Read the model definition and answer for the solid it produces. Units are mm, in the model's axes. A direction names the side the tool comes from. Round coordinates to 2 decimals unless told otherwise and drop trailing zeros. Order: outer loops, then holes, each group sorted by start corner. A loop starts at its lowest first (then second) coordinate and runs counter-clockwise, first axis right, second up. Notation, with made-up numbers: (21.5, 24) - (25.5, 24) arc R11 ccw to (25.5, 44) - close; hole circle Ø6 at (18.25, 7.5). An arc over 180 degrees is marked (long way). Answer as a JSON object with one key per item and string values. Group by question number.
Q1. A tool of negligible diameter and unlimited length cuts with its end or side. For faces 1 (the flat face through (34, 1, -5.5)), 2 (the cylindrical face through (-52.2, 1.5, 9.4)), from which of +Z, -Z, +X, -X, +Y, -Y can it reach the whole face along a straight path? Write none if from no direction.
Q2. A cutting plane is placed at C-C on z = 8.5. Count the separate pieces of the cut face and the enclosed holes in it, and give its area (3 significant figures).
Q3. Consider line 1 (X direction, y = 1.5, z = 0); line 2 (Z direction, x = 0, y = 1); line 3 (X direction, y = 0.4, z = 1). Determine where each line is inside the solid, lowest interval first.
Q4. Given pin 1 Ø5 at (x, z) = (-17, 8.5) entering from +Y; pin 2 Ø1.5 at (y, z) = (1, -12) entering from -X, each flat-ended and moving along its own axis, determine where each tip first touches the part or whether it passes through.
Q5. A cutting plane is placed at A-A on z = 0. Determine the outline of the cut face in (x, y).
Q6. A cutting plane is placed at B-B on x = 51. Determine the outline of the cut face in (y, z), and give its area (3 significant figures).
Q7. The mould has two halves that part along Z. Classify faces 3 (the cylindrical face through (0, 1, 10)), 4 (the flat face through (-17, 1, -5.5)), 5 (the flat face through (-1, 0, 3)), 6 (the cylindrical face through (15.8, 1.5, 9.4)): pulls with the +Z half, pulls with the -Z half, needs draft (parallel to the pull), parting line crosses it, or undercut.
```python
from build123d import *

# Parameters (mm, degrees)
SKETCH1_R           = 1.5
BOSS_EXTRUDE1_DEPTH = 3


with BuildPart() as part:
    # Sketch1 → Boss-Extrude1 (new body)
    with BuildSketch(Plane(origin=(0, 0, 0), x_dir=(1, 0, 0), z_dir=(0, 1, 0))):
        with BuildLine():
            Line((70, 15.5), (58.5, 15.5))
            ThreePointArc((58.5, 15.5), (57.085786438, 14.914213562), (56.5, 13.5))
            Line((56.5, 13.5), (56.5, 7.5))
            ThreePointArc((56.5, 7.5), (55.914213562, 6.085786438), (54.5, 5.5))
            Line((54.5, 5.5), (47.5, 5.5))
            ThreePointArc((47.5, 5.5), (46.085786438, 6.085786438), (45.5, 7.5))
            Line((45.5, 7.5), (45.5, 13.5))
            ThreePointArc((45.5, 13.5), (44.914213562, 14.914213562), (43.5, 15.5))
            Line((43.5, 15.5), (41.5, 15.5))
            ThreePointArc((41.5, 15.5), (40.085786438, 14.914213562), (39.5, 13.5))
            Line((39.5, 13.5), (39.5, 7.5))
            ThreePointArc((39.5, 7.5), (38.914213562, 6.085786438), (37.5, 5.5))
            Line((37.5, 5.5), (30.5, 5.5))
            ThreePointArc((30.5, 5.5), (29.085786438, 6.085786438), (28.5, 7.5))
            Line((28.5, 7.5), (28.5, 13.5))
            ThreePointArc((28.5, 13.5), (27.914213562, 14.914213562), (26.5, 15.5))
            Line((26.5, 15.5), (24.5, 15.5))
            ThreePointArc((24.5, 15.5), (23.085786438, 14.914213562), (22.5, 13.5))
            Line((22.5, 13.5), (22.5, 7.5))
            ThreePointArc((22.5, 7.5), (21.914213562, 6.085786438), (20.5, 5.5))
            Line((20.5, 5.5), (13.5, 5.5))
            ThreePointArc((13.5, 5.5), (12.085786438, 6.085786438), (11.5, 7.5))
            Line((11.5, 7.5), (11.5, 13.5))
            ThreePointArc((11.5, 13.5), (10.914213562, 14.914213562), (9.5, 15.5))
            Line((9.5, 15.5), (7.5, 15.5))
            ThreePointArc((7.5, 15.5), (6.085786438, 14.914213562), (5.5, 13.5))
            Line((5.5, 13.5), (5.5, 7.5))
            ThreePointArc((5.5, 7.5), (4.914213562, 6.085786438), (3.5, 5.5))
            Line((3.5, 5.5), (-3.5, 5.5))
            ThreePointArc((-3.5, 5.5), (-4.914213562, 6.085786438), (-5.5, 7.5))
            Line((-5.5, 7.5), (-5.5, 13.5))
            ThreePointArc((-5.5, 13.5), (-6.085786438, 14.914213562), (-7.5, 15.5))
            Line((-7.5, 15.5), (-9.5, 15.5))
            ThreePointArc((-9.5, 15.5), (-10.914213562, 14.914213562), (-11.5, 13.5))
            Line((-11.5, 13.5), (-11.5, 7.5))
            ThreePointArc((-11.5, 7.5), (-12.085786438, 6.085786438), (-13.5, 5.5))
            Line((-13.5, 5.5), (-20.5, 5.5))
            ThreePointArc((-20.5, 5.5), (-21.914213562, 6.085786438), (-22.5, 7.5))
            Line((-22.5, 7.5), (-22.5, 13.5))
            ThreePointArc((-22.5, 13.5), (-23.085786438, 14.914213562), (-24.5, 15.5))
            Line((-24.5, 15.5), (-26.5, 15.5))
            ThreePointArc((-26.5, 15.5), (-27.914213562, 14.914213562), (-28.5, 13.5))
            Line((-28.5, 13.5), (-28.5, 7.5))
            ThreePointArc((-28.5, 7.5), (-29.085786438, 6.085786438), (-30.5, 5.5))
            Line((-30.5, 5.5), (-37.5, 5.5))
            ThreePointArc((-37.5, 5.5), (-38.914213562, 6.085786438), (-39.5, 7.5))
            Line((-39.5, 7.5), (-39.5, 13.5))
            ThreePointArc((-39.5, 13.5), (-40.085786438, 14.914213562), (-41.5, 15.5))
            Line((-41.5, 15.5), (-43.5, 15.5))
            ThreePointArc((-43.5, 15.5), (-44.914213562, 14.914213562), (-45.5, 13.5))
            Line((-45.5, 13.5), (-45.5, 7.5))
            ThreePointArc((-45.5, 7.5), (-46.085786438, 6.085786438), (-47.5, 5.5))
            Line((-47.5, 5.5), (-54.5, 5.5))
            ThreePointArc((-54.5, 5.5), (-55.914213562, 6.085786438), (-56.5, 7.5))
            Line((-56.5, 7.5), (-56.5, 13.5))
            ThreePointArc((-56.5, 13.5), (-57.085786438, 14.914213562), (-58.5, 15.5))
            Line((-58.5, 15.5), (-70, 15.5))
            ThreePointArc((-70, 15.5), (-73.535533906, 14.035533906), (-75, 10.5))
            Line((-75, 10.5), (-75, -10.5))
            ThreePointArc((-75, -10.5), (-73.535533906, -14.035533906), (-70, -15.5))
            Line((-70, -15.5), (70, -15.5))
            ThreePointArc((70, -15.5), (73.535533906, -14.035533906), (75, -10.5))
            Line((75, -10.5), (75, 10.5))
            ThreePointArc((75, 10.5), (73.535533906, 14.035533906), (70, 15.5))
        make_face()
        with Locations((71, 0)):
            Circle(SKETCH1_R, mode=Mode.SUBTRACT)
        with Locations((-51, -8.5)):
            Circle(SKETCH1_R, mode=Mode.SUBTRACT)
        with Locations((-34, -8.5)):
            Circle(SKETCH1_R, mode=Mode.SUBTRACT)
        with Locations((-17, -8.5)):
            Circle(SKETCH1_R, mode=Mode.SUBTRACT)
        with Locations((0, -8.5)):
            Circle(SKETCH1_R, mode=Mode.SUBTRACT)
        with Locations((17, -8.5)):
            Circle(SKETCH1_R, mode=Mode.SUBTRACT)
        with Locations((34, -8.5)):
            Circle(SKETCH1_R, mode=Mode.SUBTRACT)
        with Locations((51, -8.5)):
            Circle(SKETCH1_R, mode=Mode.SUBTRACT)
        with Locations((-71, 0)):
            Circle(SKETCH1_R, mode=Mode.SUBTRACT)
    extrude(amount=BOSS_EXTRUDE1_DEPTH)


solid = part.part
```
Result set:
{
 "1": {"face 1": "-Z, +Y, -Y", "face 2": "+Y, -Y"},
 "2": {"separate pieces": "8", "enclosed holes": "0", "area": "387 mm²"},
 "3": {"line 1": "x = -75 to -72.5, -69.5 to 69.5, 72.5 to 75", "line 2": "z = -5.5 to 7, 10 to 15.5", "line 3": "x = -75 to -72.12, -69.88 to 69.88, 72.12 to 75"},
 "4": {"pin 1": "stops at y = 3", "pin 2": "stops at x = -74.94"},
 "5": {"outline": "(-75, 0) - (-72.5, 0) - (-72.5, 3) - (-75, 3) - close; (-69.5, 0) - (69.5, 0) - (69.5, 3) - (-69.5, 3) - close; (72.5, 0) - (75, 0) - (75, 3) - (72.5, 3) - close"},
 "6": {"outline": "(0, -5.5) - (3, -5.5) - (3, 7) - (0, 7) - close; (0, 10) - (3, 10) - (3, 15.5) - (0, 15.5) - close", "area": "54.0 mm²"},
 "7": {"face 3": "undercut", "face 4": "pulls with the -Z half", "face 5": "needs draft", "face 6": "undercut"}
}
